Study the drawing (mm; zero at the part's minimum x, y, z) and answer. Round coordinates to 2 decimals unless told otherwise and drop trailing zeros. Order: outer loops, then holes, each group sorted by start corner. A loop starts at its lowest first (then second) coordinate and runs counter-clockwise, first axis right, second up. Notation, with made-up numbers: (-21, 41) -> (18, 41) arc R18 cw to (18, 62) -> close; hole circle Ø2 at (-20, -21.75). An arc over 180 degrees is marked (long way). Use one line per item in the form item = value.
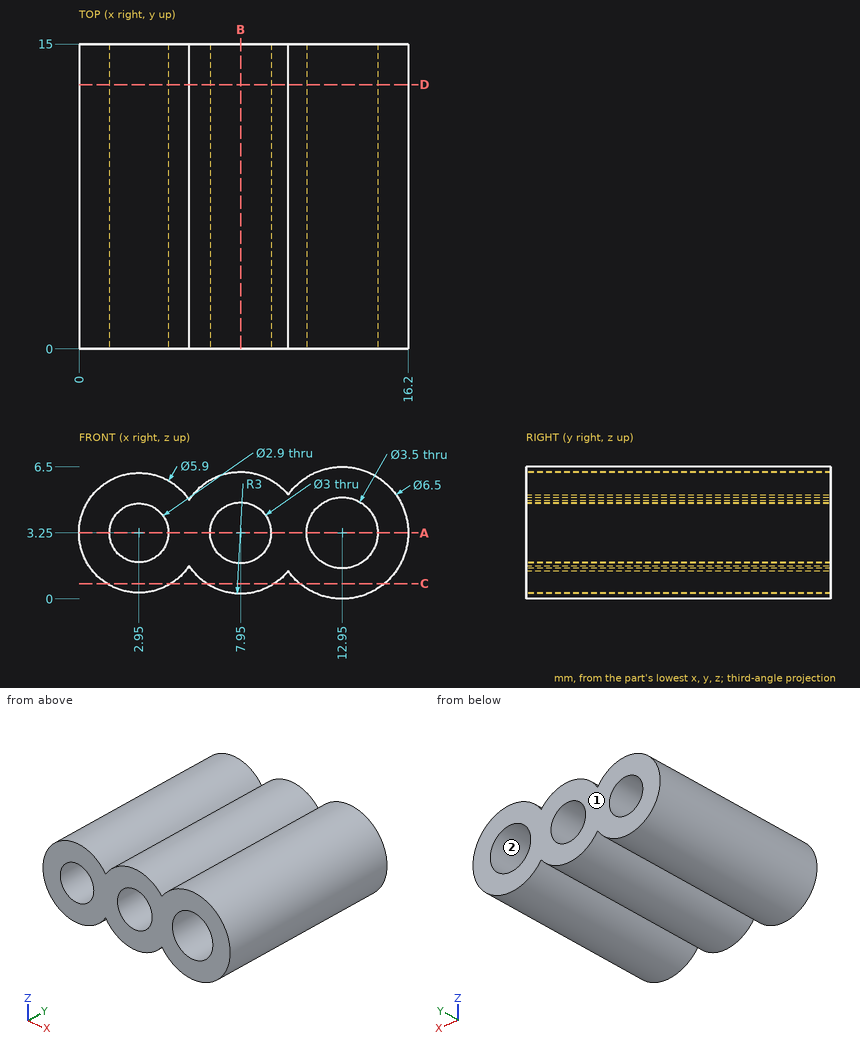
Item 1: The part is cut by section C-C, the plane z = 0.75. Give the vertices of the cut face in (x, y), and give its area (3 significant figures).
Findings:
outline = (1.38, 0) -> (4.52, 0) -> (4.52, 15) -> (1.38, 15) -> close; (6.29, 0) -> (9.61, 0) -> (9.61, 15) -> (6.29, 15) -> close; (10.87, 0) -> (15.03, 0) -> (15.03, 15) -> (10.87, 15) -> close
area = 159 mm^2
Item 2: Flat-ended cylindrical pins translate along their axes: P1, Ø2, axis at y = 8, z = 2, coming from the +X side; P2, Ø3, axis at x = 2.5, y = 10, coming from the +Z side; P3, Ø2, axis at x = 4, y = 3.5, coming from the -Z side. Find the tip coordinate at first contact, or state that the pin passes through.
Findings:
P1 = 16.19
P2 = 6.2
P3 = 0.3
Item 3: The part is cut by section D-D, the plane y = 13. Give the vertices of the cut face in (x, z).
Findings:
outline = (5.42, 1.64) arc R3 ccw to (10.29, 1.38) arc R3.25 ccw (long way) to (10.29, 5.12) arc R3 ccw to (5.42, 4.86) arc R2.95 ccw (long way) to start; hole circle Ø2.9 at (2.95, 3.25); hole circle Ø3 at (7.95, 3.25); hole circle Ø3.5 at (12.95, 3.25)
Item 4: Consider line 1 along X through (y, z) = (6.5, 3.25); line 2 along X through (y, z) = (1, 1.25); line 3 along X through (y, z) = (4, 2.5). Determine where each line is inside the solid, lowest interval first.
Findings:
line_1 = 0 to 1.5, 4.4 to 6.45, 9.45 to 11.2, 14.7 to 16.2
line_2 = 0.78 to 5.12, 5.71 to 10.19, 10.39 to 15.51
line_3 = 0.1 to 1.71, 4.19 to 6.65, 9.25 to 11.37, 14.53 to 16.11
Item 5: The part is cut by section B-B, the plane x = 7.95. Give the vertices of the cut face in (y, z), and give its area (3 significant figures).
Findings:
outline = (0, 0.25) -> (15, 0.25) -> (15, 1.75) -> (0, 1.75) -> close; (0, 4.75) -> (15, 4.75) -> (15, 6.25) -> (0, 6.25) -> close
area = 45.0 mm^2
Item 6: Determine the mould class of the marked faces 1 and 2 for opening direction X: released by +X, released by -X, zero draft, split by the parting line, or undercut.
Findings:
face_1 = zero draft
face_2 = undercut
Item 7: The part is cut by section A-A, the plane z = 3.25. Give the vertices of the cut face in (x, y).
Findings:
outline = (0, 0) -> (1.5, 0) -> (1.5, 15) -> (0, 15) -> close; (4.4, 0) -> (6.45, 0) -> (6.45, 15) -> (4.4, 15) -> close; (9.45, 0) -> (11.2, 0) -> (11.2, 15) -> (9.45, 15) -> close; (14.7, 0) -> (16.2, 0) -> (16.2, 15) -> (14.7, 15) -> close
